from build123d import *


with BuildPart() as part:
    # 草图2 → 旋转1 (revolve)
    with BuildSketch(Plane(origin=(0, 0, 0), x_dir=(0, 0, -1), z_dir=(1, 0, 0)), mode=Mode.PRIVATE) as revolve_1_sk:
        Polygon((1, 12), (2, 12), (2, 5), (1, 5), (1, 6), (0.95, 6), (0.95, 5), (-0.95, 5), (-0.95, 6), (-1, 6), (-1, 5), (-2, 5), (-2, 12), (-1, 12), (-1, 11.5), (-0.95, 11.5), (-0.95, 12), (0.95, 12), (0.95, 11.5), (1, 11.5), align=None)
    revolve(revolve_1_sk.sketch.rotate(Axis((0, 0, 2), (0, 0, -1)), 90), axis=Axis((0, 0, 2), (0, 0, -1)))


solid = part.part
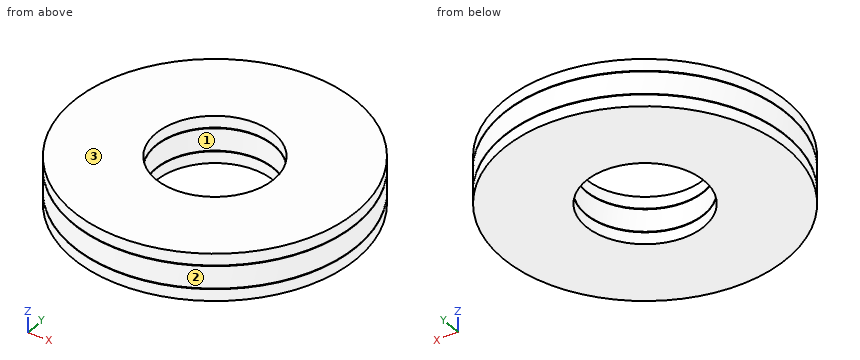
Check sheet for the modelled part. Datum: model origin and axes. Units: mm. Face numbers are marked on the shaded views. Coordinates: 2 decimals unless noted, no trailing zeros. Loops run counter-clockwise (first coordinate to the right, second up) from the corner with the lowest first, then second, coordinate; pieces in that order, holes last. Notation, with made-up numbers: (-5, -16) -> (13, -16) arc R28 cw to (13, 2) -> close; hole circle Ø5 at (70, -2.75). An arc over 180 degrees is marked (long way). Write item = value, one per line. Start each with the question number.
1. Section check A-A on z = -0.4. Record the cut outline in (x, y).
2. Section check B-B on x = -8. Record the cut outline in (y, z).
3. Draft check along X on the marked faces 1, 2 and 3. Enter one of: released by +X, released by -X, zero draft, split by the parting line, or undercut.
4. Depth check by flat-ended pin: P1, Ø6, axis at x = 0, y = 0, coming from the -Z side. Enter the tip coordinate at first touch or a pass-through.
5. Material ranges on line 1 (Y direction, x = 0, z = -1.4); line 2 (X direction, y = -4.5, z = -0.65), recorded low to high.
6. Section check C-C on y = 7.25. Record the cut outline in (x, z).
Responses:
q1.outline = circle Ø24 at (0, 0); hole circle Ø10 at (0, 0)
q2.outline = (-8.94, -2) -> (8.94, -2) -> (8.94, -1) -> (8.26, -1) -> (8.26, -0.95) -> (8.94, -0.95) -> (8.94, 0.95) -> (8.26, 0.95) -> (8.26, 1) -> (8.94, 1) -> (8.94, 2) -> (-8.94, 2) -> (-8.94, 1) -> (-8.26, 1) -> (-8.26, 0.95) -> (-8.94, 0.95) -> (-8.94, -0.95) -> (-8.26, -0.95) -> (-8.26, -1) -> (-8.94, -1) -> close
q3.face_1 = undercut
q3.face_2 = split by the parting line
q3.face_3 = zero draft
q4.P1 = through
q5.line_1 = -12 to -5, 5 to 12
q5.line_2 = -11.12 to -2.18, 2.18 to 11.12
q6.outline = (-9.56, -2) -> (9.56, -2) -> (9.56, -1) -> (8.93, -1) -> (8.93, -0.95) -> (9.56, -0.95) -> (9.56, 0.95) -> (8.93, 0.95) -> (8.93, 1) -> (9.56, 1) -> (9.56, 2) -> (-9.56, 2) -> (-9.56, 1) -> (-8.93, 1) -> (-8.93, 0.95) -> (-9.56, 0.95) -> (-9.56, -0.95) -> (-8.93, -0.95) -> (-8.93, -1) -> (-9.56, -1) -> close
